Verification items for the finished model (mm, model axes). A direction names the side the tool comes from. Coordinates: 2 decimals unless noted, no trailing zeros. Order: outer loops, then holes, each group sorted by start corner. A loop starts at its lowest first (then second) coordinate and runs counter-clockwise, first axis right, second up. Notation, with made-up numbers: M -5,22.25 L 51,22.25 A33 ccw 51,58.25 Z; hole C -16.75,56.25 d6. An arc over 180 degrees is marked long. Answer as a JSON object with one key per item and string values. Group by question number.
(1) Cross-section at D-D (z = -5.5). Enter the section's corners in (x, y), plus the area to 3 significant figures.
(2) Cross-section at A-A (z = -9.1). Enter the section's corners in (x, y), plus the area to 3 significant figures.
(3) Gauge pin test, flat ends, axial feed: pin 1 Ø5 at (x, z) = (-4, -6.5) entering from -Y; pin 2 Ø7.5 at (x, z) = (0, -5) entering from -Y; pin 3 Ø6 at (x, y) = (5.5, -14.5) entering from -Z; pin 4 Ø3.5 at (x, z) = (-13.8, -9.1) entering from -Y. Record the tip position at first contact, or that the pin passes through.
(4) Cross-section at C-C (x = 7). Enter the section's corners in (y, z), plus the area to 3 significant figures.
(5) Material ranges on line 1 (Y direction, x = -16, z = 1.25); line 2 (Y direction, x = 2.5, z = 1.5); line 3 (X direction, y = -8.5, z = -7.75), recorded low to high.
(6) Mould release check, pull along X, two halves, no side actions. Record for faces 6 (the face through (-20, 0, 1)), 7 (the face through (13.18, -6.49, -8.13)), 8 (the face through (-14.476, -15.368, 0.986)), 9 (the face through (20, 0, 1)): released by +X, released by -X, zero draft, split by the parting line, or undercut.
(7) Access from +Z, -Z, +X, -X, +Y, -Y to the whole of each face (thin tool, end or side, straight path). Record for faces 1 (the face through (0, -9, -2)), 2 (the face through (11.8, -8, -9)), 3 (the face through (-16.35, -7, -7)), 4 (the face through (0, -6, -2)), 5 (the face through (0, -7, 0)).
(8) Cross-section at B-B (y = 9). Enter the section's corners in (x, z), plus the area to 3 significant figures.
Autodesk Inventor part; units mm, degrees
ref_plane "工作平面11" through (0, -9, 0) normal (0, 1, 0) x (-1, 0, 0)
ref_plane "YZ Plane" through (0, 0, 0) normal (1, 0, 0) x (0, 1, 0)
ref_plane "XY Plane" through (0, 0, 0) normal (0, 0, 1) x (1, 0, 0)
sketch "草圖22" plane through (0, 0, 0) normal (0, 0, 1) x (1, 0, 0)
  line L0 (-20, 20) -> (20, 20)
  line L1 (20, 20) -> (20, -20)
  line L2 (20, -20) -> (-20, -20)
  line L3 (-20, -20) -> (-20, 20)
  line L4 (0, -12.2) -> (0, 0)
  line L5 (-20, 20) -> (20, -20) construction
  line L6 (20, 20) -> (-20, -20) construction
  line L7 (-16, 16) -> (16, 16) construction
  line L8 (16, 16) -> (16, -16) construction
  line L9 (16, -16) -> (-16, -16) construction
  line L10 (-16, -16) -> (-16, 16) construction
  line L11 (-16, 16) -> (16, -16) construction
  line L12 (16, 16) -> (-16, -16) construction
  circle A0 centre (-16, 16) radius 1.65
  line L13 (20, 20) -> (-10, 20)
  line L14 (-10, 20) -> (-10, -10)
  line L15 (-10, -10) -> (20, -10)
  line L16 (20, -10) -> (20, 20)
  circle A1 centre (-16, -16) radius 1.65
  circle A2 centre (16, 16) radius 1.65
  circle A3 centre (16, -16) radius 1.65
  line L17 (-10, 10) -> (10, 10)
  line L18 (10, 10) -> (10, -10)
  line L19 (10, -10) -> (-10, -10)
  line L20 (-10, -10) -> (-10, 10)
  line L21 (-20, -20) -> (20, -20)
  line L22 (20, -20) -> (20, -33.437)
  line L23 (20, -33.437) -> (-20, -33.437)
  line L24 (-20, -33.437) -> (-20, -20)
  point P0 (20, -10)
  point P1 (10, -10)
  point P2 (-10, 10)
  dimension "d118" = 40
  dimension "d119" = 16
  dimension "d120" = 3.3
  dimension "d121" = 10
  dimension "d124" = 32
  dimension "d127" = 32
extrude "擠出19" add sketch "草圖22" along normal blind 2 contours L0 L14 L15 L1 L2 L3 | L0 L1 L15 L18 L17 L14
ref_plane "工作平面5" through (0, -6, 0) normal (0, 1, 0) x (-1, 0, 0)
sketch "草圖31" plane through (0, 0, 0) normal (0, 1, 0) x (-1, 0, 0)
  line L0 (-16.35, 0) -> (16.35, 0)
  line L1 (16.35, 0) -> (16.35, -3)
  line L2 (16.35, -3) -> (-16.35, -3)
  line L3 (-16.35, -3) -> (-16.35, 0)
  line L4 (-16.35, 0) -> (16.35, -3) construction
  line L5 (16.35, 0) -> (-16.35, -3) construction
  line L6 (11.35, -3) -> (16.35, -3)
  line L7 (16.35, -3) -> (16.35, -15.2)
  line L8 (16.35, -15.2) -> (11.35, -15.2)
  line L9 (11.35, -15.2) -> (11.35, -3)
  line L10 (11.35, -3) -> (16.35, -15.2) construction
  line L11 (16.35, -3) -> (11.35, -15.2) construction
  line L12 (-11.35, -3) -> (-16.35, -3)
  line L13 (-16.35, -3) -> (-16.35, -15.2)
  line L14 (-16.35, -15.2) -> (-11.35, -15.2)
  line L15 (-11.35, -15.2) -> (-11.35, -3)
  line L16 (-11.35, -3) -> (-16.35, -15.2) construction
  line L17 (-16.35, -3) -> (-11.35, -15.2) construction
  line L18 (0, 0) -> (0, 15.4222) construction
  line L19 (-20, 0) -> (20, 0) construction
  circle A0 centre (13.8, -9.1) radius 1.15
  circle A1 centre (-13.8, -9.1) radius 1.15
  point P0 (0, -1.5)
  point P1 (13.85, -9.1)
  point P2 (-13.85, -9.1)
  dimension "d197" = 12.2
  dimension "d198" = 22.7
  dimension "d199" = 5
  dimension "d200" = 3
  dimension "d201" = 2.3
  dimension "d202" = 13.8
extrude "擠出28" add sketch "草圖31" against normal blind 3 from surface at -6
ref_plane "工作平面11" through (0, -9, 0) normal (0, 1, 0) x (-1, 0, 0)
sketch "草圖35" plane through (0, -9, 0) normal (0, 1, 0) x (-1, 0, 0)
  line L0 (-10, 0) -> (10, 0)
  line L1 (10, 0) -> (16.35, 0)
  line L2 (16.35, 0) -> (16.35, -15.2)
  line L3 (16.35, -15.2) -> (11.35, -15.2)
  line L4 (11.35, -15.2) -> (11.35, -3)
  line L5 (11.35, -3) -> (-11.35, -3)
  line L6 (-11.35, -3) -> (-11.35, -15.2)
  line L7 (-11.35, -15.2) -> (-16.35, -15.2)
  line L8 (-16.35, -15.2) -> (-16.35, 0)
  line L9 (-16.35, 0) -> (-10, 0)
  circle A0 centre (-13.8, -9.1) radius 1.15
  circle A1 centre (13.8, -9.1) radius 1.15
  line L10 (15.8, -10.7636) -> (15.8, -7.0453)
  line L11 (-11.8, -11.0386) -> (-11.8, -6.8072)
  line L12 (16.2407, -8.1997) -> (13.0206, -6.3406)
  line L13 (14.2407, -6.5362) -> (11.0206, -8.3953)
  line L14 (11.8, -7.4364) -> (11.8, -11.1547)
  line L15 (11.3593, -10.0003) -> (14.5794, -11.8594)
  line L16 (13.3593, -11.6638) -> (16.5794, -9.8047)
  line L17 (-11.1212, -8.3372) -> (-14.7856, -6.2216)
  line L18 (-13.1212, -6.3987) -> (-16.7856, -8.5143)
  line L19 (-15.8, -7.1614) -> (-15.8, -11.3928)
  line L20 (-16.4788, -9.8628) -> (-12.8144, -11.9784)
  line L21 (-14.4788, -11.8013) -> (-10.8144, -9.6857)
  point P0 (0, 0)
  point P1 (13.8, -11.4094)
  point P2 (15.8, -10.2547)
  point P3 (15.8, -7.9453)
  point P4 (13.8, -6.7906)
  point P5 (11.8, -7.9453)
  point P6 (11.8, -10.2547)
  point P7 (-13.8, -11.4094)
  point P8 (-11.8, -10.2547)
  point P9 (-11.8, -7.9453)
  point P10 (-13.8, -6.7906)
  point P11 (-15.8, -7.9453)
  point P12 (-15.8, -10.2547)
  dimension "d254" = 360
  dimension "d258" = 360
  dimension "d262" = 2
  dimension "d263" = 2
extrude "擠出32" cut sketch "草圖35" along normal blind 2 contours L18 L17 L11 L21 L20 L19 | L16 L15 L14 L13 L12 L10
properties part number "SG90_holder_1205"
Taken from the geometry:
{
 "1": {"outline": "M -16.35,-9 L -11.35,-9 L -11.35,-6 L -16.35,-6 Z; M 11.35,-9 L 16.35,-9 L 16.35,-6 L 11.35,-6 Z", "area": "30.0 mm²"},
 "2": {"outline": "M -16.35,-9 L -15.8,-9 L -15.8,-7 L -14.95,-7 L -14.95,-6 L -16.35,-6 Z; M -12.65,-7 L -11.8,-7 L -11.8,-9 L -11.35,-9 L -11.35,-6 L -12.65,-6 Z; M 11.35,-9 L 11.8,-9 L 11.8,-7 L 12.65,-7 L 12.65,-6 L 11.35,-6 Z; M 14.95,-7 L 15.8,-7 L 15.8,-9 L 16.35,-9 L 16.35,-6 L 14.95,-6 Z", "area": "9.40 mm²"},
 "3": {"pin 1": "passes through", "pin 2": "stops at y = -9", "pin 3": "stops at z = 0", "pin 4": "stops at y = -7"},
 "4": {"outline": "M -20,0 L -10,0 L -10,2 L -20,2 Z; M -9,-3 L -6,-3 L -6,0 L -9,0 Z; M 10,0 L 20,0 L 20,2 L 10,2 Z", "area": "49.0 mm²"},
 "5": {"line 1": "y = -20 to -17.65, -14.35 to 14.35, 17.65 to 20", "line 2": "y = -20 to -10, 10 to 20", "line 3": "x = -16.35 to -15.46, -12.14 to -11.35, 11.35 to 12.14, 15.46 to 16.35"},
 "6": {"face 6": "released by -X", "face 7": "undercut", "face 8": "undercut", "face 9": "released by +X"},
 "7": {"face 1": "-Z, +X, -X, -Y", "face 2": "-Y", "face 3": "-Z, -X, +Y, -Y", "face 4": "-Z, +X, -X, +Y", "face 5": "+Z"},
 "8": {"outline": "M -20,0 L -10,0 L -10,2 L -20,2 Z; M 10,0 L 20,0 L 20,2 L 10,2 Z", "area": "40.0 mm²"}
}
